The figure shows three views and two pictorial views of one solid part (mm, origin at its lowest corner). Answer the questions. A direction names the side the tool comes from. Give positions to 0.01 mm unless a question says otherwise; leave off trailing zeros. Order: outer loops, then holes, each group sorted by start corner. A loop starts at its lowest first (then second) coordinate and runs counter-clockwise, first axis right, second up. Notation, with made-up numbers: M 38.25,76 L 86.25,76 A16 cw 86.25,84 Z; hole C -19,-29 d10. An arc over 180 degrees is marked long. One line per item, written item: value.
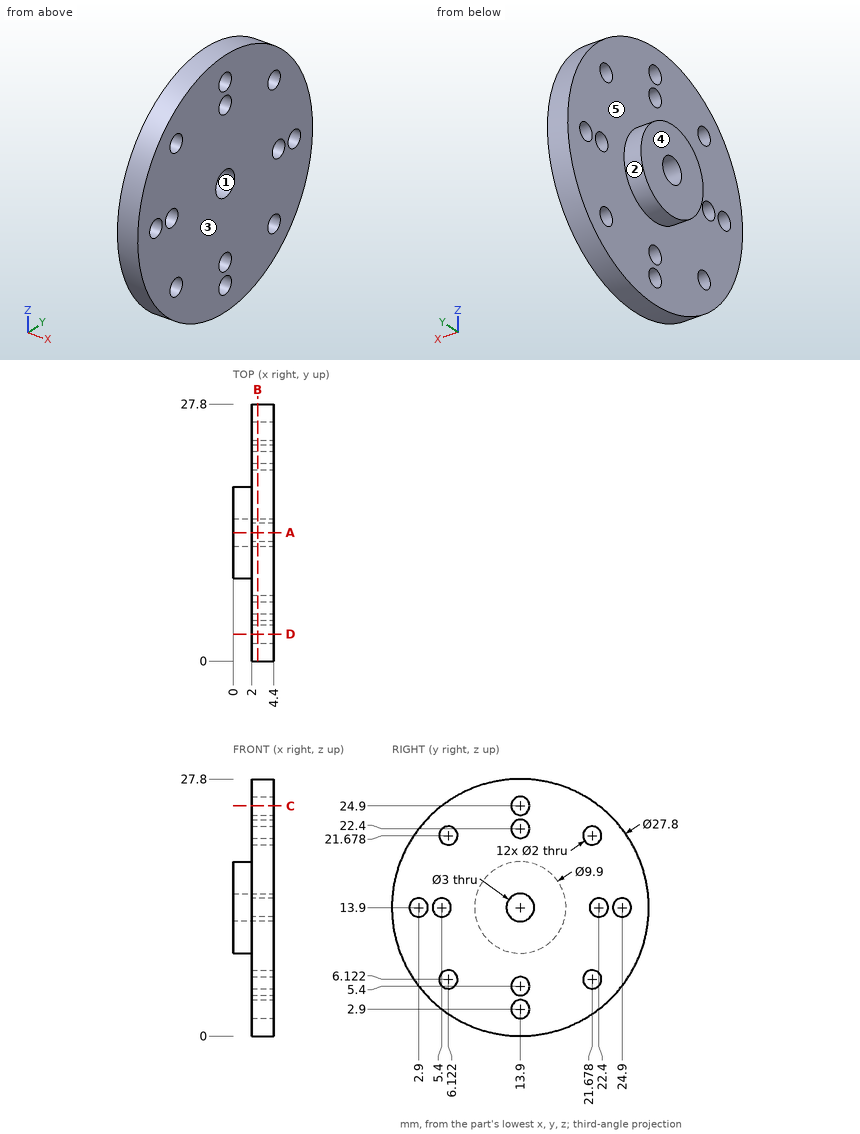
1) Find section B-B, the plane x = 2.65. Count the separate pieces of the cut face and the enclosed holes in it, plus the area to 3 significant figures.
Reported:
separate pieces: 1
enclosed holes: 13
area: 562 mm^2
2) Each of these flat-tipped pins is pushed along its axis until it touches: pin 1 Ø2 at (x, y) = (3.5, 4.5) entering from -Z (1 decimal); pin 2 Ø5 at (y, z) = (13.9, 13.9) entering from +X; pin 3 Ø2 at (x, z) = (2, 20.5) entering from +Y; pin 4 Ø2.5 at (y, z) = (13.9, 2.9) entering from -X. Where does it stop, or does it pass through?
Reported:
pin 1: stops at z = 2.8
pin 2: stops at x = 4.4
pin 3: stops at y = 26.62
pin 4: stops at x = 2
3) Which of the six approach directions +Z, -Z, +X, -X, +Y, -Y give full straight-line access (tool end or side, diameter ignored) to the marked faces 4 and 5?
Reported:
face 4: +Z, -Z, -X, +Y, -Y
face 5: -X
4) Determine the mould class of the marked faces 1, 2 and 3 for opening direction Z: +Z half, -Z half, draft (parallel to the pull), parting line (faces both ways), or undercut.
Reported:
face 1: undercut
face 2: parting line
face 3: draft
5) Find section C-C, the plane z = 24.9. Write down the section's boundary in (x, y).
Reported:
outline: M 2,5.4 L 4.4,5.4 L 4.4,12.9 L 2,12.9 Z; M 2,14.9 L 4.4,14.9 L 4.4,22.4 L 2,22.4 Z
6) Find section A-A, the plane y = 13.9. Write down the section's boundary in (x, z).
Reported:
outline: M 0,8.95 L 2,8.95 L 2,6.4 L 4.4,6.4 L 4.4,12.4 L 0,12.4 Z; M 0,15.4 L 4.4,15.4 L 4.4,21.4 L 2,21.4 L 2,18.85 L 0,18.85 Z; M 2,0 L 4.4,0 L 4.4,1.9 L 2,1.9 Z; M 2,3.9 L 4.4,3.9 L 4.4,4.4 L 2,4.4 Z; M 2,23.4 L 4.4,23.4 L 4.4,23.9 L 2,23.9 Z; M 2,25.9 L 4.4,25.9 L 4.4,27.8 L 2,27.8 Z
7) Consider probe 1 along Y at (x, z) = (2.5, 13.9); probe 2 along X at (y, z) = (11.75, 19.5); probe 3 along Z at (x, y) = (3.25, 5.4) (1 decimal). Determine where each line is inside the solid, lowest interval first.
Reported:
probe 1: y = 0 to 1.9, 3.9 to 4.4, 6.4 to 12.4, 15.4 to 21.4, 23.4 to 23.9, 25.9 to 27.8
probe 2: x = 2 to 4.4
probe 3: z = 2.9 to 5.4, 6.8 to 12.9, 14.9 to 21, 22.4 to 24.9
